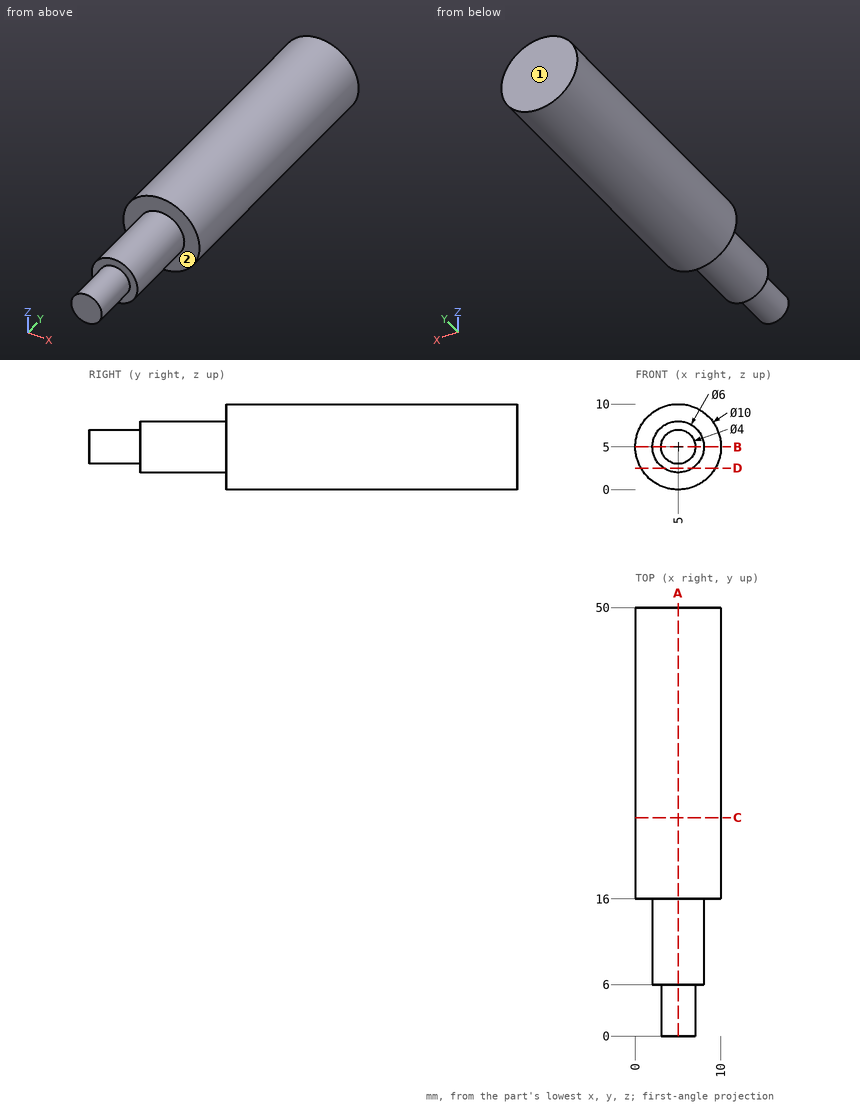
The drawing under review shows one solid part. Ordinate dimensions are in mm from its lowest x, y, z. A direction names the side the tool comes from. Coordinates: 2 decimals unless noted, no trailing zeros. Write each loop counter-clockwise with the first axis right and the second up, starting at its lowest first coordinate (ties: lowest second). Pieces come first, ordered by that corner, then holes. Notation, with made-up numbers: (87.25, 29) - (103.25, 29) arc R14 ccw to (103.25, 52) - close; hole circle Ø4 at (24, 81.5). An arc over 180 degrees is marked (long way). Answer in a Markdown table with one row per item. Add a question column.
Q1. We need section A-A, the plane x = 5. State the section outline as (y, z) points.
Q2. Tool access review of the marked faces 1 and 2: name each direction out of +Z, -Z, +X, -X, +Y, -Y from which nothing blocks a thin tool from reaching the whole face with its end or side.
Q3. We need section D-D, the plane z = 2.5. State the section outline as (x, y) points.
Q4. For probe 1 along Y at (x, z) = (2.5, 5); probe 2 along Y at (x, z) = (4, 1.25); probe 3 along Z at (x, y) = (4.75, 12.5), list the stretches that pass through material, from the lowest coordinate up.
Q5. For P1, Ø5, axis at y = 9.5, z = 7, coming from the -X side; P2, Ø2, axis at y = 17, z = 1.5, coming from the +X side; P3, Ø1, axis at x = 2.5, y = 31.5, coming from the +Z side, all flat-tipped, find the tip position at first contact; note any pin that passes through.
Q6. We need section B-B, the plane z = 5. State the section outline as (x, y) points, and give its area (3 significant figures).
Q7. We need section C-C, the plane y = 25.5. State the section outline as (x, z) points, and give its area (3 significant figures).
Answer list:
| question | item | result |
|---|---|---|
| 1 | outline | (0, 3) - (6, 3) - (6, 2) - (16, 2) - (16, 0) - (50, 0) - (50, 10) - (16, 10) - (16, 8) - (6, 8) - (6, 7) - (0, 7) - close |
| 2 | face 1 | +Z, -Z, +X, -X, +Y |
| 2 | face 2 | -Y |
| 3 | outline | (0.67, 16) - (3.34, 16) - (3.34, 6) - (6.66, 6) - (6.66, 16) - (9.33, 16) - (9.33, 50) - (0.67, 50) - close |
| 4 | probe 1 | y = 6 to 50 |
| 4 | probe 2 | y = 16 to 50 |
| 4 | probe 3 | z = 2.01 to 7.99 |
| 5 | P1 | stops at x = 2 |
| 5 | P2 | stops at x = 9.33 |
| 5 | P3 | stops at z = 9.58 |
| 6 | outline | (0, 16) - (2, 16) - (2, 6) - (3, 6) - (3, 0) - (7, 0) - (7, 6) - (8, 6) - (8, 16) - (10, 16) - (10, 50) - (0, 50) - close |
| 6 | area | 424 mm2 |
| 7 | outline | circle Ø10 at (5, 5) |
| 7 | area | 78.5 mm2 |
